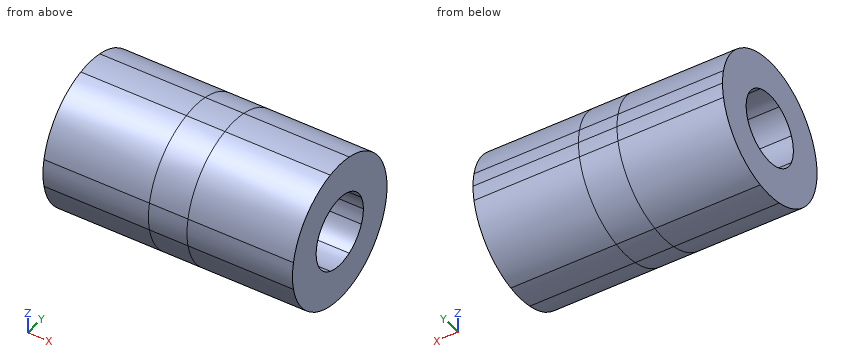
```python
from build123d import *

# Parameters (mm, degrees)
F1_DEPTH = 25.4
F2_DEPTH = 44.00509


# Not quite as in the source:
# - a pattern or mirror of a feature is missing from the dataset's text; its kind, count and spacing are read off the source's solid
# - a feature names something its author has since deleted; it is built from what else it names


with BuildPart() as f1:
    # F0 (on Right) → F1 (new body)
    with BuildSketch(Plane.YZ):
        with BuildLine():
            ThreePointArc((12.4434078933, -2.54), (12.6356891432, -1.2764638175), (12.7, 0))
            ThreePointArc((12.7, 0), (12.6356891432, 1.2764638175), (12.4434078933, 2.54))
            Line((12.4434078933, 2.54), (5.8198711326, 2.54))
            ThreePointArc((5.8198711326, 2.54), (6.2160550871, 1.2973662374), (6.35, 0))
            ThreePointArc((6.35, 0), (6.2160550871, -1.2973662374), (5.8198711326, -2.54))
            Line((5.8198711326, -2.54), (12.4434078933, -2.54))
        make_face()
        with BuildLine():
            Line((5.8198711326, 2.54), (12.4434078933, 2.54))
            ThreePointArc((12.4434078933, 2.54), (8.9802561211, 8.9802561211), (2.54, 12.4434078933))
            Line((2.54, 12.4434078933), (2.54, 5.8198711326))
            ThreePointArc((2.54, 5.8198711326), (4.4901280605, 4.4901280605), (5.8198711326, 2.54))
        make_face()
        with BuildLine():
            ThreePointArc((2.54, -12.4434078933), (8.9802561211, -8.9802561211), (12.4434078933, -2.54))
            Line((12.4434078933, -2.54), (5.8198711326, -2.54))
            ThreePointArc((5.8198711326, -2.54), (4.4901280605, -4.4901280605), (2.54, -5.8198711326))
            Line((2.54, -5.8198711326), (2.54, -12.4434078933))
        make_face()
        with BuildLine():
            Line((2.54, 5.8198711326), (2.54, 12.4434078933))
            ThreePointArc((2.54, 12.4434078933), (0, 12.7), (-2.54, 12.4434078933))
            Line((-2.54, 12.4434078933), (-2.54, 5.8198711326))
            ThreePointArc((-2.54, 5.8198711326), (0, 6.35), (2.54, 5.8198711326))
        make_face()
        with BuildLine():
            ThreePointArc((-2.54, -12.4434078933), (0, -12.7), (2.54, -12.4434078933))
            Line((2.54, -12.4434078933), (2.54, -5.8198711326))
            ThreePointArc((2.54, -5.8198711326), (0, -6.35), (-2.54, -5.8198711326))
            Line((-2.54, -5.8198711326), (-2.54, -12.4434078933))
        make_face()
        with BuildLine():
            Line((-2.54, 5.8198711326), (-2.54, 12.4434078933))
            ThreePointArc((-2.54, 12.4434078933), (-8.9802561211, 8.9802561211), (-12.4434078933, 2.54))
            Line((-12.4434078933, 2.54), (-5.8198711326, 2.54))
            ThreePointArc((-5.8198711326, 2.54), (-4.4901280605, 4.4901280605), (-2.54, 5.8198711326))
        make_face()
        with BuildLine():
            ThreePointArc((-12.4434078933, -2.54), (-8.9802561211, -8.9802561211), (-2.54, -12.4434078933))
            Line((-2.54, -12.4434078933), (-2.54, -5.8198711326))
            ThreePointArc((-2.54, -5.8198711326), (-4.4901280605, -4.4901280605), (-5.8198711326, -2.54))
            Line((-5.8198711326, -2.54), (-12.4434078933, -2.54))
        make_face()
        with BuildLine():
            Line((-5.8198711326, 2.54), (-12.4434078933, 2.54))
            ThreePointArc((-12.4434078933, 2.54), (-12.7, 0), (-12.4434078933, -2.54))
            Line((-12.4434078933, -2.54), (-5.8198711326, -2.54))
            ThreePointArc((-5.8198711326, -2.54), (-6.35, 0), (-5.8198711326, 2.54))
        make_face()
    extrude(amount=F1_DEPTH)

    # F1_copies: F1 across plane


with BuildPart() as f1_1:
    add(f1.part)
    add(f1.part.mirror(Plane(origin=(22.002045, 0, 0), x_dir=(0, 0, 1), z_dir=(1, 0, 0))))

    # F0 (on Right) → F2 (join, through all)
    with BuildSketch(Plane.YZ):
        with BuildLine():
            ThreePointArc((12.4434078933, -2.54), (12.6356891432, -1.2764638175), (12.7, 0))
            ThreePointArc((12.7, 0), (12.6356891432, 1.2764638175), (12.4434078933, 2.54))
            Line((12.4434078933, 2.54), (5.8198711326, 2.54))
            ThreePointArc((5.8198711326, 2.54), (6.2160550871, 1.2973662374), (6.35, 0))
            ThreePointArc((6.35, 0), (6.2160550871, -1.2973662374), (5.8198711326, -2.54))
            Line((5.8198711326, -2.54), (12.4434078933, -2.54))
        make_face()
        with BuildLine():
            Line((5.8198711326, 2.54), (12.4434078933, 2.54))
            ThreePointArc((12.4434078933, 2.54), (8.9802561211, 8.9802561211), (2.54, 12.4434078933))
            Line((2.54, 12.4434078933), (2.54, 5.8198711326))
            ThreePointArc((2.54, 5.8198711326), (4.4901280605, 4.4901280605), (5.8198711326, 2.54))
        make_face()
        with BuildLine():
            ThreePointArc((2.54, -12.4434078933), (8.9802561211, -8.9802561211), (12.4434078933, -2.54))
            Line((12.4434078933, -2.54), (5.8198711326, -2.54))
            ThreePointArc((5.8198711326, -2.54), (4.4901280605, -4.4901280605), (2.54, -5.8198711326))
            Line((2.54, -5.8198711326), (2.54, -12.4434078933))
        make_face()
        with BuildLine():
            Line((2.54, 5.8198711326), (2.54, 12.4434078933))
            ThreePointArc((2.54, 12.4434078933), (0, 12.7), (-2.54, 12.4434078933))
            Line((-2.54, 12.4434078933), (-2.54, 5.8198711326))
            ThreePointArc((-2.54, 5.8198711326), (0, 6.35), (2.54, 5.8198711326))
        make_face()
        with BuildLine():
            ThreePointArc((-2.54, -12.4434078933), (0, -12.7), (2.54, -12.4434078933))
            Line((2.54, -12.4434078933), (2.54, -5.8198711326))
            ThreePointArc((2.54, -5.8198711326), (0, -6.35), (-2.54, -5.8198711326))
            Line((-2.54, -5.8198711326), (-2.54, -12.4434078933))
        make_face()
        with BuildLine():
            Line((-2.54, 5.8198711326), (-2.54, 12.4434078933))
            ThreePointArc((-2.54, 12.4434078933), (-8.9802561211, 8.9802561211), (-12.4434078933, 2.54))
            Line((-12.4434078933, 2.54), (-5.8198711326, 2.54))
            ThreePointArc((-5.8198711326, 2.54), (-4.4901280605, 4.4901280605), (-2.54, 5.8198711326))
        make_face()
        with BuildLine():
            ThreePointArc((-12.4434078933, -2.54), (-8.9802561211, -8.9802561211), (-2.54, -12.4434078933))
            Line((-2.54, -12.4434078933), (-2.54, -5.8198711326))
            ThreePointArc((-2.54, -5.8198711326), (-4.4901280605, -4.4901280605), (-5.8198711326, -2.54))
            Line((-5.8198711326, -2.54), (-12.4434078933, -2.54))
        make_face()
        with BuildLine():
            Line((-5.8198711326, 2.54), (-12.4434078933, 2.54))
            ThreePointArc((-12.4434078933, 2.54), (-12.7, 0), (-12.4434078933, -2.54))
            Line((-12.4434078933, -2.54), (-5.8198711326, -2.54))
            ThreePointArc((-5.8198711326, -2.54), (-6.35, 0), (-5.8198711326, 2.54))
        make_face()
    extrude(amount=F2_DEPTH)


solid = f1_1.part
```
CAD build for the part. Positions are in the model's coordinates, mm. Round coordinates to 2 decimals unless told otherwise and drop trailing zeros. Write each loop counter-clockwise with the first axis right and the second up, starting at its lowest first coordinate (ties: lowest second). Pieces come first, ordered by that corner, then holes. Notation, with made-up numbers: (83, -8.75) -> (93, -8.75) arc R36 ccw to (93, 28.25) -> close; hole circle Ø7 at (-37.75, 35.5). An arc over 180 degrees is marked (long way). Answer in a Markdown table with one row per item. Add a question column.
Item 1: Drill centre lines: line 1 (Y direction, x = 40, z = -3.5); line 2 (Y direction, x = 25.5, z = 2.25); line 3 (Z direction, x = 12, y = -5.25). Where is each one in solid material? Low to high. Write a range as from..to.
Item 2: Saw through at A-A, the plane y = 0. Write the cut outline in (x, z), then the cut area to 3 significant figures.
Item 3: Drop flat-ended pins along their axis: pin 1 Ø2 at (x, y) = (32.5, 3.5) entering from -Z; pin 2 Ø2 at (x, z) = (7.5, 6.5) entering from +Y; pin 3 Ø3 at (x, z) = (37.5, -7.5) entering from -Y. Give the stop position or say it passes through.
Item 4: Saw through at B-B, the plane x = 20. Write the cut outline in (y, z).
Item 5: Saw through at C-C, the plane z = 1. Write the cut outline in (x, y), then the cut area to 3 significant figures.
Item 6: Saw through at D-D, the plane y = -11. Write the cut outline in (x, z), then the cut area to 3 significant figures.
Findings below:
| question | item | result |
|---|---|---|
| 1 | line 1 | y = -12.21..-5.3, 5.3..12.21 |
| 1 | line 2 | y = -12.5..-5.94, 5.94..12.5 |
| 1 | line 3 | z = -11.56..-3.57, 3.57..11.56 |
| 2 | outline | (0, -12.7) -> (44.01, -12.7) -> (44.01, -6.35) -> (0, -6.35) -> close; (0, 6.35) -> (44.01, 6.35) -> (44.01, 12.7) -> (0, 12.7) -> close |
| 2 | area | 559 mm^2 |
| 3 | pin 1 | stops at z = -12.45 |
| 3 | pin 2 | stops at y = 11.45 |
| 3 | pin 3 | stops at y = -11.19 |
| 4 | outline | circle Ø25.4 at (0, 0); hole circle Ø12.7 at (0, 0) |
| 5 | outline | (0, -12.66) -> (44.01, -12.66) -> (44.01, -6.27) -> (0, -6.27) -> close; (0, 6.27) -> (44.01, 6.27) -> (44.01, 12.66) -> (0, 12.66) -> close |
| 5 | area | 562 mm^2 |
| 6 | outline | (0, -6.35) -> (44.01, -6.35) -> (44.01, 6.35) -> (0, 6.35) -> close |
| 6 | area | 559 mm^2 |
